Verification items for the finished model (mm, model axes). A direction names the side the tool comes from. Give positions to 0.01 mm unless a question says otherwise; leave off trailing zeros. Loops run counter-clockwise (first coordinate to the right, second up) from the corner with the lowest first, then second, coordinate; pieces in that order, holes last. Notation, with made-up numbers: (-10.75, 80.25) -> (-3.75, 80.25) arc R3 ccw to (-3.75, 85.25) -> close; hole circle Ø2 at (-25.5, 89.5). An arc over 180 degrees is marked (long way). Answer in a Markdown table with one row per item. Add a question column.
Q1. Section check C-C on y = 22. Enter the section's corners in (x, z).
Q2. Release check for a two-part mould opening along X. For faces 4 (the face through (50.036, 8.944, -49.587)), 5 (the face through (-8, 23, -37)), 6 (the face through (40, 14.5, 21.4)), 7 (the face through (-44, 5, -45)) record: pulls with the +X half, pulls with the -X half, needs draft (parallel to the pull), parting line crosses it, or undercut.
Q3. Section check B-B on x = -17. Enter the section's corners in (y, z).
Q4. Material ranges on probe 1 along Z at (x, y) = (38, 6.5); probe 2 along Z at (x, y) = (8.5, 3); probe 3 along Z at (x, y) = (5.5, 26.5), recorded low to high.
Q5. Set-up check for faces 1 (the face through (1.116, 6.972, -36.774)), 2 (the face through (44.854, 8.902, -20.137)), 3 (the face through (12, 4, -14)): record each of +Z, -Z, +X, -X, +Y, -Y from which the full face is reachable in a straight line by a thin tool's end or side.
Q6. Gauge pin test, flat ends, axial feed: P1, Ø0.9, axis at x = 8, y = 2.5, coming from the +Z side; P2, Ø5, axis at x = -12.5, z = -22, coming from the +Y side; P3, Ø6.5, axis at y = 4, z = -10.5, coming from the +X side. Record the tip position at first contact, or that the pin passes through.
Q7. Section check A-A on z = -45. Enter the section's corners in (x, y), and give its area (3 significant figures).
Q8. Section check D-D on z = -14. Enter the section's corners in (x, y).
```python
from build123d import *

# Parameters (mm, degrees)
SKETCH1_W            = 77
SKETCH1_H            = 77
SKETCH1_W_2          = 70
SKETCH1_H_2          = 70
BOSS_EXTRUDE1_DEPTH  = 30
SKETCH2_W            = 77
SKETCH2_H            = 77
BOSS_EXTRUDE2_DEPTH  = 2
SKETCH3_R            = 2.6
SKETCH3_R_2          = 0.75
BOSS_EXTRUDE3_DEPTH  = 20
FILLET1_R            = 3
BOSS_EXTRUDE8_DEPTH  = 6
SKETCH15_R           = 5.15
CUT_EXTRUDE2_DEPTH   = 3.5
BOSS_EXTRUDE9_DEPTH  = 8
CHAMFER1_SIZE        = 3
CHAMFER2_SIZE        = 3
SKETCH18_W           = 25
SKETCH18_H           = 32
BOSS_EXTRUDE10_DEPTH = 2
SKETCH19_R           = 0.75
CUT_EXTRUDE3_DEPTH   = 83.003048724
SKETCH20_R           = 5.15
CUT_EXTRUDE4_DEPTH   = 3.5
CHAMFER3_SIZE        = 3
CHAMFER3_SIZE_2      = 20
SKETCH21_W           = 15
SKETCH21_H           = 10
CUT_EXTRUDE5_DEPTH   = 3.5


with BuildPart() as part:
    # Sketch1 → Boss-Extrude1 (new body)
    with BuildSketch(Plane(origin=(0, 0, 0), x_dir=(1, 0, 0), z_dir=(0, 1, 0))):
        Rectangle(SKETCH1_W, SKETCH1_H)
        Rectangle(SKETCH1_W_2, SKETCH1_H_2, mode=Mode.SUBTRACT)
    extrude(amount=BOSS_EXTRUDE1_DEPTH)

    # Sketch2 → Boss-Extrude2 (add)
    with BuildSketch(Plane.XZ):
        Rectangle(SKETCH2_W, SKETCH2_H)
    extrude(amount=BOSS_EXTRUDE2_DEPTH)

    # Sketch3 → Boss-Extrude3 (add)
    # profile 1 of 4: a face of its own
    with BuildSketch(Plane(origin=(0, 0, 0), x_dir=(1, 0, 0), z_dir=(0, 1, 0))):
        with Locations(Location((28, 28, 0), (0, 0, 90))):
            Circle(SKETCH3_R)
        with Locations(Location((28, 28, 0), (0, 0, 270))):
            Circle(SKETCH3_R_2, mode=Mode.SUBTRACT)
    # profile 2 of 4: a face of its own
    with BuildSketch(Plane(origin=(0, 0, 0), x_dir=(1, 0, 0), z_dir=(0, 1, 0))):
        with Locations(Location((28, -28, 0), (0, 0, 90))):
            Circle(SKETCH3_R)
        with Locations(Location((28, -28, 0), (0, 0, 90))):
            Circle(SKETCH3_R_2, mode=Mode.SUBTRACT)
    # profile 3 of 4: a face of its own
    with BuildSketch(Plane(origin=(0, 0, 0), x_dir=(1, 0, 0), z_dir=(0, 1, 0))):
        with Locations(Location((-28, -28, 0), (0, 0, 90))):
            Circle(SKETCH3_R)
        with Locations(Location((-28, -28, 0), (0, 0, 270))):
            Circle(SKETCH3_R_2, mode=Mode.SUBTRACT)
    # profile 4 of 4: a face of its own
    with BuildSketch(Plane(origin=(0, 0, 0), x_dir=(1, 0, 0), z_dir=(0, 1, 0))):
        with Locations(Location((-28, 28, 0), (0, 0, 90))):
            Circle(SKETCH3_R)
        with Locations(Location((-28, 28, 0), (0, 0, 90))):
            Circle(SKETCH3_R_2, mode=Mode.SUBTRACT)
    extrude(amount=BOSS_EXTRUDE3_DEPTH)

    # Fillet1
    fillet1_edges = [part.edges().sort_by_distance(p)[0] for p in [
        (-38.5, -2, 0),
        (0, -2, -38.5),
        (38.5, -2, 0),
        (0, -2, 38.5),
    ]]
    fillet(fillet1_edges, radius=FILLET1_R)

    # Sketch11 → Boss-Extrude8 (add)
    with BuildSketch(Plane(origin=(0, 0, 0), x_dir=(1, 0, 0), z_dir=(0, 1, 0))):
        Polygon((-7, 31), (-7, 29), (-10, 29), (-10, -1), (10, -1), (10, 29), (7, 29), (7, 31), (12, 31), (12, -3), (-12, -3), (-12, 31), align=None)
    extrude(amount=BOSS_EXTRUDE8_DEPTH)

    # Sketch15 → Cut-Extrude2 (cut)
    with BuildSketch(Plane(origin=(0, 0, -38.5), x_dir=(-1, 0, 0), z_dir=(0, 0, -1))):
        with Locations((0, 12)):
            Circle(SKETCH15_R)
    extrude(amount=-CUT_EXTRUDE2_DEPTH, mode=Mode.SUBTRACT)

    # Sketch17 → Boss-Extrude9 (add)
    with BuildSketch(Plane(origin=(0, 5, 0), x_dir=(-1, 0, 0), z_dir=(0, -1, 0))):
        with BuildLine():
            Line((38.5, 22.5), (38.5, 11.5))
            Line((38.5, 11.5), (51.388037435, 29.018518519))
            ThreePointArc((51.388037435, 29.018518519), (49.813708499, 49.813708499), (29.018518519, 51.388037435))
            Line((29.018518519, 51.388037435), (11.5, 38.5))
            Line((11.5, 38.5), (22.5, 38.5))
            Line((22.5, 38.5), (30.5, 38.5))
            ThreePointArc((30.5, 38.5), (44.156854249, 44.156854249), (38.5, 30.5))
            Line((38.5, 30.5), (38.5, 22.5))
        make_face()
        with BuildLine():
            Line((-38.5, 30.5), (-38.5, 22.5))
            Line((-38.5, 22.5), (-38.5, 11.5))
            Line((-38.5, 11.5), (-51.388037435, 29.018518519))
            ThreePointArc((-51.388037435, 29.018518519), (-49.813708499, 49.813708499), (-29.018518519, 51.388037435))
            Line((-29.018518519, 51.388037435), (-11.5, 38.5))
            Line((-11.5, 38.5), (-22.5, 38.5))
            Line((-22.5, 38.5), (-30.5, 38.5))
            ThreePointArc((-30.5, 38.5), (-44.156854249, 44.156854249), (-38.5, 30.5))
        make_face()
        with BuildLine():
            Line((38.5, -30.5), (38.5, -22.5))
            Line((38.5, -22.5), (38.5, -11.5))
            Line((38.5, -11.5), (51.388037435, -29.018518519))
            ThreePointArc((51.388037435, -29.018518519), (49.813708499, -49.813708499), (29.018518519, -51.388037435))
            Line((29.018518519, -51.388037435), (11.5, -38.5))
            Line((11.5, -38.5), (22.5, -38.5))
            Line((22.5, -38.5), (30.5, -38.5))
            ThreePointArc((30.5, -38.5), (44.156854249, -44.156854249), (38.5, -30.5))
        make_face()
        with BuildLine():
            Line((-22.5, -38.5), (-30.5, -38.5))
            ThreePointArc((-30.5, -38.5), (-44.156854249, -44.156854249), (-38.5, -30.5))
            Line((-38.5, -30.5), (-38.5, -22.5))
            Line((-38.5, -22.5), (-38.5, -11.5))
            Line((-38.5, -11.5), (-51.388037435, -29.018518519))
            ThreePointArc((-51.388037435, -29.018518519), (-49.813708499, -49.813708499), (-29.018518519, -51.388037435))
            Line((-29.018518519, -51.388037435), (-11.5, -38.5))
            Line((-11.5, -38.5), (-22.5, -38.5))
        make_face()
    extrude(amount=-BOSS_EXTRUDE9_DEPTH)

    # Chamfer1
    chamfer1_edges = [part.edges().sort_by_distance(p)[0] for p in [
        (-38.5, 13, -21),
        (-21, 13, -38.5),
        (-21, 5, -38.5),
        (-38.5, 5, -21),
        (38.5, 13, -21),
        (21, 13, -38.5),
        (21, 5, -38.5),
        (38.5, 5, -21),
        (-38.5, 13, 21),
        (-21, 13, 38.5),
        (-21, 5, 38.5),
        (-38.5, 5, 21),
        (21, 13, 38.5),
        (38.5, 13, 21),
        (38.5, 5, 21),
        (21, 5, 38.5),
    ]]
    chamfer(chamfer1_edges, length=CHAMFER1_SIZE)

    # Chamfer2
    chamfer2_edges = [part.edges().sort_by_distance(p)[0] for p in [
        (-12, 0, -14),
        (12, 0, -14),
    ]]
    chamfer(chamfer2_edges, length=CHAMFER2_SIZE)

    # Sketch18 → Boss-Extrude10 (add)
    with BuildSketch(Plane(origin=(0, 0, 0), x_dir=(1, 0, 0), z_dir=(0, 1, 0))):
        with Locations((0, -19)):
            Rectangle(SKETCH18_W, SKETCH18_H)
    extrude(amount=BOSS_EXTRUDE10_DEPTH)

    # Sketch19 → Cut-Extrude3 (cut, through all)
    with BuildSketch(Plane(origin=(0, 2, 0), x_dir=(1, 0, 0), z_dir=(0, 1, 0))):
        with Locations(Location((0, -6, 0), (0, 0, 270))):
            Circle(SKETCH19_R)
        with Locations(Location((0, -32, 0), (0, 0, 270))):
            Circle(SKETCH19_R)
    extrude(amount=-CUT_EXTRUDE3_DEPTH, mode=Mode.SUBTRACT)

    # Sketch20 → Cut-Extrude4 (cut)
    with BuildSketch(Plane.ZY.offset(38.5)):
        with Locations((0, 12)):
            Circle(SKETCH20_R)
    extrude(amount=-CUT_EXTRUDE4_DEPTH, mode=Mode.SUBTRACT)

    # Chamfer3
    # the kernel refuses this chamfer: 20, 3 mm, written as the material it adds along each edge
    with BuildSketch(Plane(origin=(28, 0, -28), x_dir=(0, 0, -1), z_dir=(1, 0, 0))) as chamfer3_piece_1_section:
        Polygon((2.6 + CHAMFER3_SIZE, 0), (2.6, CHAMFER3_SIZE_2), (2.6, 0), align=None)
    chamfer3_piece_1 = revolve(axis=Axis((28, 0, -28), (0, 1, 0)), mode=Mode.PRIVATE)
    chamfer3_piece_1 = split(chamfer3_piece_1, bisect_by=Plane(origin=(28, 20, -23.934343061), z_dir=(0, -1, 0)), keep=Keep.TOP, mode=Mode.PRIVATE)
    add(chamfer3_piece_1)
    with BuildSketch(Plane(origin=(28, 0, 28), x_dir=(0, 0, -1), z_dir=(1, 0, 0))) as chamfer3_piece_2_section:
        Polygon((2.6 + CHAMFER3_SIZE, 0), (2.6, CHAMFER3_SIZE_2), (2.6, 0), align=None)
    chamfer3_piece_2 = revolve(axis=Axis((28, 0, 28), (0, 1, 0)), mode=Mode.PRIVATE)
    chamfer3_piece_2 = split(chamfer3_piece_2, bisect_by=Plane(origin=(28, 20, 32.065656938), z_dir=(0, -1, 0)), keep=Keep.TOP, mode=Mode.PRIVATE)
    add(chamfer3_piece_2)
    with BuildSketch(Plane(origin=(-28, 0, 28), x_dir=(0, 0, -1), z_dir=(1, 0, 0))) as chamfer3_piece_3_section:
        Polygon((2.6 + CHAMFER3_SIZE, 0), (2.6, CHAMFER3_SIZE_2), (2.6, 0), align=None)
    chamfer3_piece_3 = revolve(axis=Axis((-28, 0, 28), (0, 1, 0)), mode=Mode.PRIVATE)
    chamfer3_piece_3 = split(chamfer3_piece_3, bisect_by=Plane(origin=(-28, 20, 32.065656938), z_dir=(0, -1, 0)), keep=Keep.TOP, mode=Mode.PRIVATE)
    add(chamfer3_piece_3)
    with BuildSketch(Plane(origin=(-28, 0, -28), x_dir=(0, 0, -1), z_dir=(1, 0, 0))) as chamfer3_piece_4_section:
        Polygon((2.6 + CHAMFER3_SIZE, 0), (2.6, CHAMFER3_SIZE_2), (2.6, 0), align=None)
    chamfer3_piece_4 = revolve(axis=Axis((-28, 0, -28), (0, 1, 0)), mode=Mode.PRIVATE)
    chamfer3_piece_4 = split(chamfer3_piece_4, bisect_by=Plane(origin=(-28, 20, -23.934343061), z_dir=(0, -1, 0)), keep=Keep.TOP, mode=Mode.PRIVATE)
    add(chamfer3_piece_4)

    # Sketch21 → Cut-Extrude5 (cut)
    with BuildSketch(Plane.XY.offset(-35)):
        with Locations((-15.5, 23)):
            Rectangle(SKETCH21_W, SKETCH21_H)
    extrude(amount=-CUT_EXTRUDE5_DEPTH, mode=Mode.SUBTRACT)


solid = part.part
```
Taken from the geometry:
| question | item | result |
|---|---|---|
| 1 | outline | (-38.5, -38.5) -> (-23, -38.5) -> (-23, -35) -> (-35, -35) -> (-35, 35) -> (35, 35) -> (35, -35) -> (-8, -35) -> (-8, -38.5) -> (38.5, -38.5) -> (38.5, 38.5) -> (-38.5, 38.5) -> close |
| 2 | face 4 | undercut |
| 2 | face 5 | undercut |
| 2 | face 6 | pulls with the +X half |
| 2 | face 7 | needs draft |
| 3 | outline | (-2, -35.5) arc R3 ccw to (1, -38.5) -> (2, -38.5) -> (5, -41.5) -> (5, -42.55) -> (13, -42.55) -> (13, -41.5) -> (16, -38.5) -> (18, -38.5) -> (18, -35) -> (0, -35) -> (0, 35) -> (30, 35) -> (30, 38.5) -> (16, 38.5) -> (13, 41.5) -> (13, 42.55) -> (5, 42.55) -> (5, 41.5) -> (2, 38.5) -> (1, 38.5) arc R3 ccw to (-2, 35.5) -> close; (28, -38.5) -> (30, -38.5) -> (30, -35) -> (28, -35) -> close |
| 4 | probe 1 | z = -54.49 to -46.48, -38.5 to 38.5, 46.48 to 54.49 |
| 4 | probe 2 | z = -38.5 to -35, -31 to -29, 1 to 3, 35 to 38.5 |
| 4 | probe 3 | z = -38.5 to -35, 35 to 38.5 |
| 5 | face 1 | -Z |
| 5 | face 2 | +X, +Y, -Y |
| 5 | face 3 | +Y |
| 6 | P1 | stops at z = 38.5 |
| 6 | P2 | stops at y = 6 |
| 6 | P3 | stops at x = 40.16 |
| 7 | outline | (-53.12, 5) -> (-43.16, 5) -> (-43.16, 13) -> (-53.12, 13) -> close; (-33.84, 5) -> (-20.34, 5) -> (-20.34, 13) -> (-33.84, 13) -> close; (20.34, 5) -> (33.84, 5) -> (33.84, 13) -> (20.34, 13) -> close; (43.16, 5) -> (53.12, 5) -> (53.12, 13) -> (43.16, 13) -> close |
| 7 | area | 375 mm² |
| 8 | outline | (-40.34, 3.84) -> (-38.5, 2) -> (-38.5, 1) arc R3 ccw to (-35.5, -2) -> (35.5, -2) arc R3 ccw to (38.5, 1) -> (38.5, 2) -> (40.34, 3.84) -> (40.34, 14.16) -> (38.5, 16) -> (38.5, 30) -> (35, 30) -> (35, 0) -> (15, 0) -> (12, 3) -> (12, 6) -> (10, 6) -> (10, 0) -> (-10, 0) -> (-10, 6) -> (-12, 6) -> (-12, 3) -> (-15, 0) -> (-35, 0) -> (-35, 30) -> (-38.5, 30) -> (-38.5, 16) -> (-40.34, 14.16) -> close |
